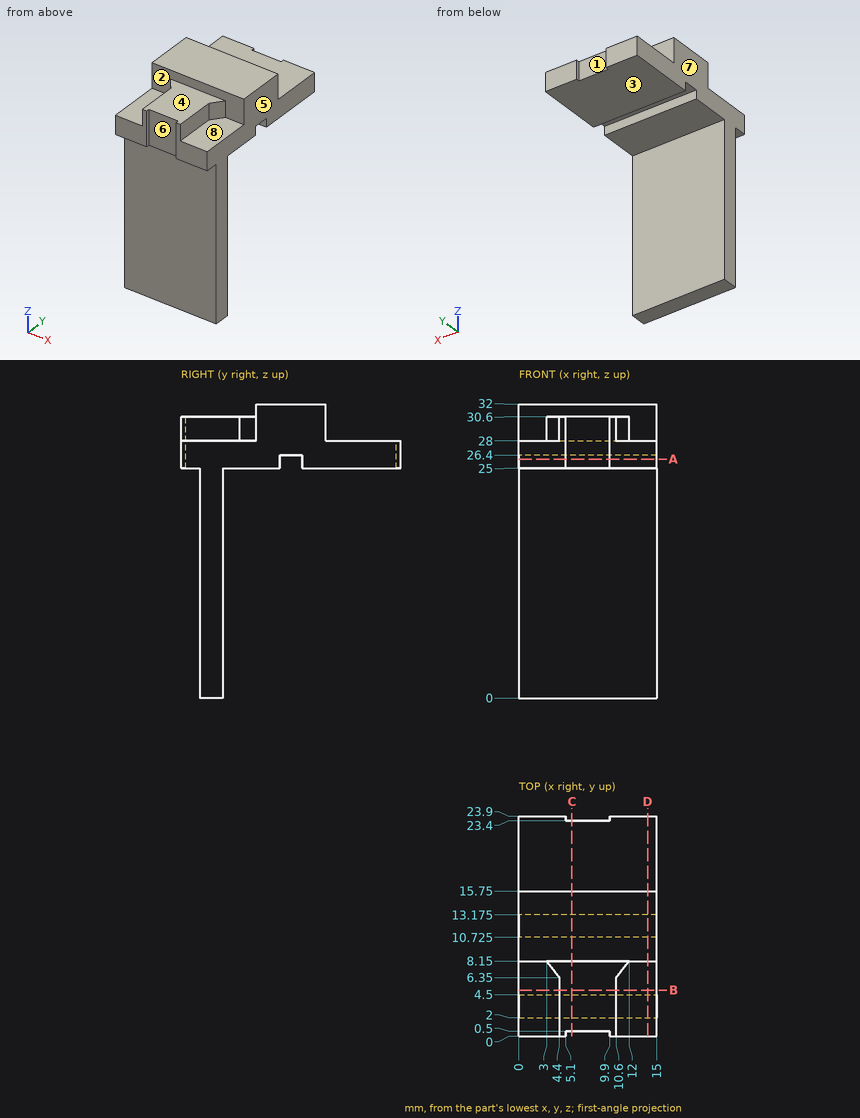
Study the drawing (mm; zero at the part's minimum x, y, z) and answer. A direction names the side the tool comes from. Round coordinates to 2 decimals unless told otherwise and drop trailing zeros. Write each loop counter-clockwise with the first axis right and the second up, starting at its lowest first coordinate (ties: lowest second). Pieces come first, ordered by that corner, then holes.
1) A cutting plane is placed at B-B (y = 5). Give the vertices of the cut face in (x, z), plus the area to 3 significant figures.
2) A cutting plane is placed at D-D (x = 14). Give the vertices of the cut face in (y, z) (3 decimals), plus the area to 3 significant figures.
3) A cutting plane is placed at A-A (z = 26). Give the vertices of the cut face in (x, y) (3 decimals), plus the area to 3 significant figures.
4) The mould has two halves that part along X. Classify the marked faces 5, 6, 7 and 8: pulls with the +X half, pulls with the -X half, needs draft (parallel to the pull), parting line crosses it, or undercut.
5) A tool of negligible diameter and unlimited length cuts with its end or side. For the marked faces 1, 2, 3 and 4, from which of +Z, -Z, +X, -X, +Y, -Y can it reach the whole face along a straight path? Write none if from no direction.
6) Straight lines are drawn through the part: line 1 (Z direction, x = 12, y = 8); line 2 (Z direction, x = 10, y = 15.5); line 3 (Y direction, x = 12.75, z = 19.5). For each, find the intervals that lie inside material, in ascending order.
7) Given pin 1 Ø1.9 at (x, y) = (5.5, 8.5) entering from -Z; pin 2 Ø3 at (x, z) = (8, 30.5) entering from -Y; pin 3 Ø3.5 at (x, y) = (3, 5) entering from +Z; pin 4 Ø6 at (y, z) = (8, 5) entering from +X, each flat-ended and moving along its own axis, determine where each tip first touches the part or whether it passes through.
8) A cutting plane is placed at C-C (x = 5.75). Give the vertices of the cut face in (y, z) (3 decimals), plus the area to 3 significant figures.
Completed:
1. outline: (0, 25) - (15, 25) - (15, 28) - (10.6, 28) - (10.6, 30.6) - (4.4, 30.6) - (4.4, 28) - (0, 28) - close
1. area: 61.1 mm2
2. outline: (0, 25) - (2, 25) - (2, 0) - (4.5, 0) - (4.5, 25) - (10.725, 25) - (10.725, 26.4) - (13.175, 26.4) - (13.175, 25) - (23.9, 25) - (23.9, 28) - (15.75, 28) - (15.75, 32) - (8.15, 32) - (8.15, 28) - (0, 28) - close
2. area: 161 mm2
3. outline: (0, 0) - (5.1, 0) - (5.1, 0.5) - (9.9, 0.5) - (9.9, 0) - (15, 0) - (15, 10.725) - (0, 10.725) - close; (0, 13.175) - (15, 13.175) - (15, 23.9) - (9.9, 23.9) - (9.9, 23.4) - (5.1, 23.4) - (5.1, 23.9) - (0, 23.9) - close
3. area: 317 mm2
4. face 5: pulls with the +X half
4. face 6: undercut
4. face 7: pulls with the -X half
4. face 8: needs draft
5. face 1: +Z, -Z, +Y
5. face 2: +Z, -Y
5. face 3: -Z, +X, -X, +Y
5. face 4: +Z, +X, -X, -Y
6. line 1: z = 25 to 28
6. line 2: z = 25 to 32
6. line 3: y = 2 to 4.5
7. pin 1: stops at z = 25
7. pin 2: stops at y = 0.5
7. pin 3: stops at z = 30.6
7. pin 4: passes through
8. outline: (0.5, 25) - (2, 25) - (2, 0) - (4.5, 0) - (4.5, 25) - (10.725, 25) - (10.725, 26.4) - (13.175, 26.4) - (13.175, 25) - (23.4, 25) - (23.4, 28) - (15.75, 28) - (15.75, 32) - (8.15, 32) - (8.15, 30.6) - (0.5, 30.6) - close
8. area: 178 mm2
